from build123d import *

# Parameters (mm, degrees)
BOSS_EXTRUDE1_DEPTH     = 3
SKETCH2_W               = 3
SKETCH2_H               = 18
SKETCH2_W_2             = 17.666666666
SKETCH2_H_2             = 3
SKETCH2_W_3             = 17.666666667
SKETCH2_W_4             = 9.5
SKETCH2_W_5             = 20
CUT_EXTRUDE1_DEPTH      = 1
CUT_EXTRUDE1_DEPTH_BACK = 4
SKETCH3_W               = 3.2
SKETCH3_H               = 10.5
SKETCH3_W_2             = 5.2
SKETCH3_H_2             = 2.5
CUT_EXTRUDE2_DEPTH      = 1
CUT_EXTRUDE2_DEPTH_BACK = 4
FILLET1_R               = 7.5
FILLET2_R               = 2.5
SKETCH4_W               = 3
SKETCH4_H               = 10.5
CUT_EXTRUDE3_DEPTH      = 4
CUT_EXTRUDE3_DEPTH_BACK = 1


with BuildPart() as part:
    # Sketch1 → Boss-Extrude1 (new body)
    with BuildSketch(Plane.XY):
        Polygon((-130, 33), (130, 33), (130, -33), (114.5, -33), (114.5, 0), (79.5, 0), (79.5, -33), (-79.5, -33), (-79.5, 0), (-114.5, 0), (-114.5, -33), (-130, -33), align=None)
    extrude(amount=BOSS_EXTRUDE1_DEPTH)

    # Sketch2 → Cut-Extrude1 (cut, two sides)
    with BuildSketch(Plane.XY.offset(3)) as cut_extrude1_sk:
        with Locations((-128.5, 21)):
            Rectangle(SKETCH2_W, SKETCH2_H)
        with Locations((-128.5, -15)):
            Rectangle(SKETCH2_W, SKETCH2_H)
        with Locations((-53, -28.5)):
            Rectangle(SKETCH2_W_2, SKETCH2_H_2)
        with Locations((-17.666666666, -28.5)):
            Rectangle(SKETCH2_W_3, SKETCH2_H_2)
        with Locations((17.666666666, -28.5)):
            Rectangle(SKETCH2_W_3, SKETCH2_H_2)
        with Locations((53, -28.5)):
            Rectangle(SKETCH2_W_2, SKETCH2_H_2)
        with Locations((122.25, -28.5)):
            Rectangle(SKETCH2_W_4, SKETCH2_H_2)
        with Locations((128.5, -15)):
            Rectangle(SKETCH2_W, SKETCH2_H)
        with Locations((128.5, 21)):
            Rectangle(SKETCH2_W, SKETCH2_H)
        Polygon((130, 33), (110, 33), (110, 30), (127, 30), (130, 30), align=None)
        with Locations((80, 31.5)):
            Rectangle(SKETCH2_W_5, SKETCH2_H_2)
        with Locations((40, 31.5)):
            Rectangle(SKETCH2_W_5, SKETCH2_H_2)
        with Locations((-40, 31.5)):
            Rectangle(SKETCH2_W_5, SKETCH2_H_2)
        with Locations((-80, 31.5)):
            Rectangle(SKETCH2_W_5, SKETCH2_H_2)
        with Locations((0, 31.5)):
            Rectangle(SKETCH2_W_5, SKETCH2_H_2)
        with Locations((-120, 31.5)):
            Rectangle(SKETCH2_W_5, SKETCH2_H_2)
        with Locations((-122.25, -28.5)):
            Rectangle(SKETCH2_W_4, SKETCH2_H_2)
    extrude(amount=CUT_EXTRUDE1_DEPTH, mode=Mode.SUBTRACT)
    extrude(cut_extrude1_sk.sketch, amount=-CUT_EXTRUDE1_DEPTH_BACK, mode=Mode.SUBTRACT)

    # Sketch3 → Cut-Extrude2 (cut, two sides)
    with BuildSketch(Plane.XY.offset(3)) as cut_extrude2_sk:
        with Locations((-60, 27.75)):
            Rectangle(SKETCH3_W, SKETCH3_H)
        with Locations((60, 27.75)):
            Rectangle(SKETCH3_W, SKETCH3_H)
        with Locations((-60, 28.575)):
            Rectangle(SKETCH3_W_2, SKETCH3_H_2)
        with Locations((60, 28.575)):
            Rectangle(SKETCH3_W_2, SKETCH3_H_2)
    extrude(amount=CUT_EXTRUDE2_DEPTH, mode=Mode.SUBTRACT)
    extrude(cut_extrude2_sk.sketch, amount=-CUT_EXTRUDE2_DEPTH_BACK, mode=Mode.SUBTRACT)

    # Fillet1
    fillet1_edges = [part.edges().sort_by_distance(p)[0] for p in [
        (114.5, 0, 1.5),
        (79.5, 0, 1.5),
        (-79.5, 0, 1.5),
        (-114.5, 0, 1.5),
    ]]
    fillet(fillet1_edges, radius=FILLET1_R)

    # Fillet2
    fillet2_edges = [part.edges().sort_by_distance(p)[0] for p in [
        (114.5, -33, 1.5),
        (79.5, -33, 1.5),
        (-79.5, -33, 1.5),
        (-114.5, -33, 1.5),
    ]]
    fillet(fillet2_edges, radius=FILLET2_R)

    # Sketch4 → Cut-Extrude3 (cut, two sides)
    with BuildSketch(Plane.XY) as cut_extrude3_sk:
        with Locations((-111.15, 24.75)):
            Rectangle(SKETCH4_W, SKETCH4_H)
        with Locations((111.15, 24.75)):
            Rectangle(SKETCH4_W, SKETCH4_H)
    extrude(amount=CUT_EXTRUDE3_DEPTH, mode=Mode.SUBTRACT)
    extrude(cut_extrude3_sk.sketch, amount=-CUT_EXTRUDE3_DEPTH_BACK, mode=Mode.SUBTRACT)


solid = part.part
Work out the finished part from the listing and answer in its coordinate system (mm). A direction names the side the tool comes from. Coordinates: 2 decimals unless noted, no trailing zeros. Write each loop counter-clockwise with the first axis right and the second up, starting at its lowest first coordinate (ties: lowest second). Pieces come first, ordered by that corner, then holes. Notation, with made-up numbers: M -21,28.5 L 34,28.5 A19 ccw 34,54.5 Z; hole C -2.75,45.25 d7. An arc over 180 degrees is marked long. Answer as CSV lines item,"result". Start each with the question number.
Item 1: Section A-A on x = 21 is taken. Write down the section's boundary in (y, z).
Item 2: Section C-C on z = 0.6 is taken. Give the number of separate pieces and of enclosed holes in the cut face, and give its area (3 significant figures).
Item 3: Consider L1, parallel to X at y = -9.5, z = 2.2; L2, parallel to X at y = 26.5, z = 1.25; L3, parallel to Y at x = 20, z = 0.8. Determine where each line is inside the solid, lowest interval first.
Item 4: Section B-B on y = -18 is taken. Write down the section's boundary in (x, z), and give its area (3 significant figures).
Item 5: A tool of negligible diameter and unlimited length cuts with its end or side. For faces 3 (the face through (2, 8, 0)), 4 (the face through (-81.755, -2.139, 1.521)), from which of +Z, -Z, +X, -X, +Y, -Y can it reach the whole face along a straight path? Write none if from no direction.
Item 6: Flat-ended cylindrical pins translate along their axes: P1, Ø10, axis at x = -17, y = -25.5, coming from the -Z side; P2, Ø1.5, axis at y = 27, z = 2, coming from the +X side. Find the tip coordinate at first contact, or state that the pin passes through.
Item 7: Determine the mould class of faces 1 (the face through (81.639, -2.255, 1.521)), 2 (the face through (2, 8, 3)) for opening direction X: released by +X, released by -X, zero draft, split by the parting line, or undercut.
Checks:
1,outline,"M -33,0 L -30,0 L -30,3 L -33,3 Z; M -27,0 L 33,0 L 33,3 L -27,3 Z"
2,separate pieces,"1"
2,enclosed holes,"6"
2,area,"13,800 mm²"
3,L1,"x = -127 to -114.5, -79.5 to 79.5, 114.5 to 127"
3,L2,"x = -127 to -112.65, -109.65 to -61.6, -58.4 to 58.4, 61.6 to 109.65, 112.65 to 127"
3,L3,"y = -33 to -30, -27 to 33"
4,outline,"M -127,0 L -114.5,0 L -114.5,3 L -127,3 Z; M -79.5,0 L 79.5,0 L 79.5,3 L -79.5,3 Z; M 114.5,0 L 127,0 L 127,3 L 114.5,3 Z"
4,area,"552 mm²"
5,face 3,"-Z, +X, -X, +Y, -Y"
5,face 4,"+Z, -Z, -Y"
6,P1,"stops at z = 0"
6,P2,"stops at x = 127"
7,face 1,"undercut"
7,face 2,"zero draft"
